Input: part model. Units: mm. Frame: model coordinates. Coordinates: 2 decimals unless noted, no trailing zeros. Write each loop counter-clockwise with the first axis right and the second up, starting at its lowest first coordinate (ties: lowest second). Pieces come first, ordered by that corner, then holes.
1) Pin query (flat end, axial travel): pin 1 Ø4 at (x, z) = (52.28, -90.54) entering from +Y; pin 2 Ø6 at (y, z) = (6.5, -56) entering from -X; pin 3 Ø4 at (x, y) = (61.5, 10.5) entering from +Z; pin 4 Ø3 at (y, z) = (9.5, -49.5) entering from -X. Return the tip coordinate at first contact, or that it passes through.
2) Section query A-A (z = -95). Output: boundary loops of the cut face in (x, y), then the cut area to 3 significant figures.
3) Section query C-C (x = -46). Output: boundary loops of the cut face in (y, z), then the cut area to 3 significant figures.
4) Line query: L1, parallel to Z at x = -0.5, y = 5.5; L2, parallel to X at y = 7, z = 30; L3, parallel to Z at x = 33, y = 11.5. Output: solid intervals per line, ascending.
5) Section query B-B (y = 5.75). State how many separate pieces and enclosed holes the cut face has, then the cut area to 3 significant figures.
from build123d import *

# Parameters (mm, degrees)
SKETCH1_R           = 1.65
BOSS_EXTRUDE1_DEPTH = 12.7
FILLET1_R           = 5


with BuildPart() as part:
    # Sketch1 → Boss-Extrude1 (new body)
    with BuildSketch(Plane(origin=(0, 0, 0), x_dir=(1, 0, 0), z_dir=(0, 1, 0))):
        with BuildLine():
            ThreePointArc((-111.234035703, -19.613561667), (-112.95, 0), (-111.234035703, 19.613561667))
            ThreePointArc((-111.234035703, 19.613561667), (-109.13025705, 22.87401705), (-105.327953741, 23.647931427))
            ThreePointArc((-105.327953741, 23.647931427), (0, 107.95), (105.327953741, 23.647931427))
            ThreePointArc((105.327953741, 23.647931427), (109.13025705, 22.87401705), (111.234035703, 19.613561667))
            ThreePointArc((111.234035703, 19.613561667), (112.95, 0), (111.234035703, -19.613561667))
            ThreePointArc((111.234035703, -19.613561667), (109.13025705, -22.87401705), (105.327953741, -23.647931427))
            ThreePointArc((105.327953741, -23.647931427), (0, -107.95), (-105.327953741, -23.647931427))
            ThreePointArc((-105.327953741, -23.647931427), (-109.13025705, -22.87401705), (-111.234035703, -19.613561667))
        make_face()
        with Locations(Location((0, 104.55, 0), (0, 0, 270))):
            Circle(SKETCH1_R, mode=Mode.SUBTRACT)
        with Locations(Location((52.275, 90.542955966, 0), (0, 0, 270))):
            Circle(SKETCH1_R, mode=Mode.SUBTRACT)
        with Locations(Location((90.542955966, 52.275, 0), (0, 0, 270))):
            Circle(SKETCH1_R, mode=Mode.SUBTRACT)
        with Locations(Location((104.55, 0, 0), (0, 0, 270))):
            Circle(SKETCH1_R, mode=Mode.SUBTRACT)
        with Locations(Location((90.542955966, -52.275, 0), (0, 0, 270))):
            Circle(SKETCH1_R, mode=Mode.SUBTRACT)
        with Locations(Location((52.275, -90.542955966, 0), (0, 0, 270))):
            Circle(SKETCH1_R, mode=Mode.SUBTRACT)
        with Locations(Location((0, -104.55, 0), (0, 0, 270))):
            Circle(SKETCH1_R, mode=Mode.SUBTRACT)
        with Locations(Location((-52.275, -90.542955966, 0), (0, 0, 270))):
            Circle(SKETCH1_R, mode=Mode.SUBTRACT)
        with Locations(Location((-90.542955966, -52.275, 0), (0, 0, 270))):
            Circle(SKETCH1_R, mode=Mode.SUBTRACT)
        with Locations(Location((-104.55, 0, 0), (0, 0, 270))):
            Circle(SKETCH1_R, mode=Mode.SUBTRACT)
        with Locations(Location((-90.542955966, 52.275, 0), (0, 0, 270))):
            Circle(SKETCH1_R, mode=Mode.SUBTRACT)
        with Locations(Location((-52.275, 90.542955966, 0), (0, 0, 270))):
            Circle(SKETCH1_R, mode=Mode.SUBTRACT)
    extrude(amount=BOSS_EXTRUDE1_DEPTH)

    # Fillet1
    fillet1_edges = [part.edges().sort_by_distance(p)[0] for p in [
        (-105.327953741, 6.35, -23.647931427),
        (105.327953741, 6.35, -23.647931427),
        (105.327953741, 6.35, 23.647931427),
        (-105.327953741, 6.35, 23.647931427),
    ]]
    fillet(fillet1_edges, radius=FILLET1_R)


solid = part.part
Answer:
1. pin 1: stops at y = 12.7
1. pin 2: stops at x = -94.04
1. pin 3: stops at z = 90.07
1. pin 4: stops at x = -96.69
2. outline: (-51.27, 0) - (51.27, 0) - (51.27, 12.7) - (-51.27, 12.7) - close
2. area: 1,300 mm2
3. outline: (0, -97.66) - (12.7, -97.66) - (12.7, 97.66) - (0, 97.66) - close
3. area: 2,480 mm2
4. L1: z = -107.95 to -106.12, -102.98 to 102.98, 106.12 to 107.95
4. L2: x = -103.7 to 103.7
4. L3: z = -102.78 to 102.78
5. separate pieces: 1
5. enclosed holes: 12
5. area: 37,000 mm2
